The model under review builds one solid part; all positions refer to its coordinate system, in mm. A direction names the side the tool comes from. Give positions to 0.01 mm unless a question says otherwise; leave off trailing zeros. Loops run counter-clockwise (first coordinate to the right, second up) from the corner with the lowest first, then second, coordinate; pieces in that order, holes last. Notation, with made-up numbers: M 46,45 L 86,45 A15 ccw 86,74 Z; hole C 84,13 d9. An arc over 180 degrees is marked long. One line per item, written item: value. Start each with the question number.
Q1. We need section B-B on x = 1. Write out the cut boundary in (y, z), plus the area to 3 significant figures.
Q2. Mouldability with a two-part tool opening along X and no side actions: class faces 1 (the face through (4.95, 3, 0)), 2 (the face through (1, 0.2, 1.1)), 3 (the face through (4, 0, 0)) as released by +X, released by -X, zero draft, split by the parting line, or undercut.
Q3. For faces 4 (the face through (3, 4, 1.85)), 5 (the face through (-4, 0, 0)), 6 (the face through (4, 1, 1.85)), list the 3-axis set-ups (+Z, -Z, +X, -X, +Y, -Y) from which the entire face can be reached by the end or side of a thin tool; tool diameter is ignored.
Q4. We need section C-C on z = 2. Write out the cut boundary in (x, y), plus the area to 3 significant figures.
Q5. To check wall thickness, follow line 1 along Z through (x, y) = (-3, 5); line 2 along Z through (x, y) = (2.5, 2); line 3 along Z through (x, y) = (-2.25, 2.25). State the ranges of each line that lie inside material, in increasing order. Write a range as from..to.
Q6. We need section D-D on y = 4.5. Give the number of separate pieces and of enclosed holes in the cut face, plus the area to 4 significant figures.
Q7. We need section A-A on y = -0.5. Write out the cut boundary in (x, z), plus the area to 3 significant figures.
Q8. For pin 1 (0.6 mm diameter, centred on x = -3, y = -2, fed in from -Z); pin 2 (0.5 mm diameter, centred on x = 3, z = 1.5, fed in from -Y); pin 3 (2 mm diameter, centred on y = -0.5, z = 1.5, fed in from -X); pin 4 (1.5 mm diameter, centred on x = 2.5, z = -0.5, fed in from +Y), all flat-tipped, find the tip position at first contact; note any pin that passes through.
```python
from build123d import *

# Parameters (mm, degrees)
SKETCH_1_W                                 = 4.95
SKETCH_1_H                                 = 4.7
EXTRUDE_1_DEPTH                            = 1.73
EXTRUDE_2_DEPTH                            = 4.27
CUT_EXTRUDE_1_DEPTH                        = 1.5
CUT_EXTRUDE_3_DEPTH                        = 4.45
SKETCH_4_W                                 = 1.05
SKETCH_4_H                                 = 4
SKETCH_4_W_2                               = 2.45
SKETCH_4_H_2                               = 4.27
CUT_EXTRUDE_2_DEPTH                        = 0.5
CUT_EXTRUDE_4_DEPTH                        = 0.5
EXTRUDE_START                              = -5
SKETCH_5_W                                 = 0.5
SKETCH_5_H                                 = 0.5
EXTRUDE_3_DEPTH                            = 8.9
CHAMFER_1_SIZE                             = 0.1
CHAMFER_1_SIZE2                            = 0.567128182
CHAMFER_1_PART_2_SIZE                      = 0.1
CHAMFER_1_PART_2_SIZE2                     = 0.567128182
PATTERN_LINEAR_1_COUNT                     = 4
PATTERN_LINEAR_1_PITCH                     = 2
CHAMFER_1_OF_PATTERN_LINEAR_1_SIZE2        = 0.1
CHAMFER_1_OF_PATTERN_LINEAR_1_SIZE         = 0.567128182
CHAMFER_1_PART_2_OF_PATTERN_LINEAR_1_SIZE2 = 0.1
CHAMFER_1_PART_2_OF_PATTERN_LINEAR_1_SIZE  = 0.567128182


with BuildPart() as part:
    # Эскиз1 → Бобышка-Вытянуть1 (new body)
    with BuildSketch(Plane(origin=(0, 0, 0), x_dir=(1, 0, 0), z_dir=(0, 1, 0))):
        with Locations((-2.475, 0)):
            Rectangle(SKETCH_1_W, SKETCH_1_H)
    extrude_1 = extrude(amount=EXTRUDE_1_DEPTH)

    # Эскиз2 → Бобышка-Вытянуть2 (add)
    with BuildSketch(Plane(origin=(0, 1.73, 0), x_dir=(1, 0, 0), z_dir=(0, 1, 0))):
        Polygon((0, 2.35), (-4.95, 2.35), (-4.95, -2.35), (0, -2.35), (0, -1.85), (-4.45, -1.85), (-4.45, 1.85), (0, 1.85), align=None)
    extrude_2 = extrude(amount=EXTRUDE_2_DEPTH)

    # Эскиз3 → Вырез-Вытянуть1 (cut, through all)
    with BuildSketch(Plane(origin=(-4.45, 0, 0), x_dir=(0, 0, -1), z_dir=(1, 0, 0))):
        with BuildLine():
            Line((-1.35, 6), (-0.35, 6))
            Line((-0.35, 6), (-0.35, 4.3))
            ThreePointArc((-0.35, 4.3), (-0.437867966, 4.087867966), (-0.65, 4))
            Line((-0.65, 4), (-1.05, 4))
            ThreePointArc((-1.05, 4), (-1.262132034, 4.087867966), (-1.35, 4.3))
            Line((-1.35, 4.3), (-1.35, 6))
        make_face()
    cut_extrude_1 = extrude(amount=-CUT_EXTRUDE_1_DEPTH, mode=Mode.SUBTRACT)

    # Эскиз8 → Вырез-Вытянуть3 (cut)
    with BuildSketch(Plane(origin=(0, 0, 0), x_dir=(0, 0, -1), z_dir=(1, 0, 0))):
        Polygon((0, 1.73), (0.55, 1.23), (1.85, 1.23), (1.85, 1.73), align=None)
    cut_extrude_3 = extrude(amount=-CUT_EXTRUDE_3_DEPTH, mode=Mode.SUBTRACT)

    # Эскиз4 → Вырез-Вытянуть2 (cut)
    with BuildSketch(Plane.XY.offset(2.35)):
        with Locations((-3.925, 2)):
            Rectangle(SKETCH_4_W, SKETCH_4_H)
        with Locations((-1.225, 3.865)):
            Rectangle(SKETCH_4_W_2, SKETCH_4_H_2)
    cut_extrude_2 = extrude(amount=-CUT_EXTRUDE_2_DEPTH, mode=Mode.SUBTRACT)

    # Зеркальное отражение1: Бобышка-Вытянуть1, Бобышка-Вытянуть2, Вырез-Вытянуть1, Вырез-Вытянуть3, Вырез-Вытянуть2 across plane
    add(extrude_1.mirror(Plane(origin=(0, 0, 0), x_dir=(0, 0, 1), z_dir=(1, 0, 0))))
    add(extrude_2.mirror(Plane(origin=(0, 0, 0), x_dir=(0, 0, 1), z_dir=(1, 0, 0))))
    add(cut_extrude_1.mirror(Plane(origin=(0, 0, 0), x_dir=(0, 0, 1), z_dir=(1, 0, 0))), mode=Mode.SUBTRACT)
    add(cut_extrude_3.mirror(Plane(origin=(0, 0, 0), x_dir=(0, 0, 1), z_dir=(1, 0, 0))), mode=Mode.SUBTRACT)
    add(cut_extrude_2.mirror(Plane(origin=(0, 0, 0), x_dir=(0, 0, 1), z_dir=(1, 0, 0))), mode=Mode.SUBTRACT)

    # Эскиз9 → Вырез-Вытянуть4 (cut, symmetric)
    with BuildSketch(Plane.ZY.offset(3)):
        Polygon((2.35, 0), (-2.35, 0), (-2.35, 0.5), (-0.05, 0.2), (2.35, 0.2), align=None)
    cut_extrude_4 = extrude(amount=CUT_EXTRUDE_4_DEPTH, both=True, mode=Mode.SUBTRACT)

    # Эскиз5 → Бобышка-Вытянуть3 (add)
    with BuildSketch(Plane(origin=(0, 1.73, 0), x_dir=(1, 0, 0), z_dir=(0, 1, 0)).offset(EXTRUDE_START)):
        with Locations((-3, -0.65)):
            Rectangle(SKETCH_5_W, SKETCH_5_H)
    extrude_3 = extrude(amount=EXTRUDE_3_DEPTH)

    # Фаска1
    chamfer_1_edges = [part.edges().sort_by_distance(p)[0] for p in [
        (-3.25, 5.63, 0.65),
        (-3, 5.63, 0.4),
        (-2.75, 5.63, 0.65),
        (-3, 5.63, 0.9),
    ]]
    chamfer_1_side = [part.faces().sort_by_distance(p)[0] for p in [
        (-3, 5.63, 0.65),
    ]]
    chamfer(chamfer_1_edges, length=CHAMFER_1_SIZE, length2=CHAMFER_1_SIZE2, reference=chamfer_1_side[0])

    # Фаска1 part 2
    chamfer_1_part_2_edges = [part.edges().sort_by_distance(p)[0] for p in [
        (-3.25, -3.27, 0.65),
        (-3, -3.27, 0.4),
        (-2.75, -3.27, 0.65),
        (-3, -3.27, 0.9),
    ]]
    chamfer_1_part_2_side = [part.faces().sort_by_distance(p)[0] for p in [
        (-3, -3.27, 0.65),
    ]]
    chamfer(chamfer_1_part_2_edges, length=CHAMFER_1_PART_2_SIZE, length2=CHAMFER_1_PART_2_SIZE2, reference=chamfer_1_part_2_side[0])

    # Линейный массив1: Вырез-Вытянуть4, Бобышка-Вытянуть3 ×4
    with Locations(*[(i * PATTERN_LINEAR_1_PITCH, 0, 0) for i in range(1, PATTERN_LINEAR_1_COUNT)]):
        add(cut_extrude_4, mode=Mode.SUBTRACT)
        add(extrude_3)

    # Фаска1 of Линейный массив1
    chamfer_1_of_pattern_linear_1_edges = [part.edges().sort_by_distance(p)[0] for p in [
        (-1.25, 5.63, 0.65),
        (-1, 5.63, 0.4),
        (-0.75, 5.63, 0.65),
        (-1, 5.63, 0.9),
        (0.75, 5.63, 0.65),
        (1, 5.63, 0.4),
        (1.25, 5.63, 0.65),
        (1, 5.63, 0.9),
        (2.75, 5.63, 0.65),
        (3, 5.63, 0.4),
        (3.25, 5.63, 0.65),
        (3, 5.63, 0.9),
    ]]
    chamfer(chamfer_1_of_pattern_linear_1_edges, length=CHAMFER_1_OF_PATTERN_LINEAR_1_SIZE, length2=CHAMFER_1_OF_PATTERN_LINEAR_1_SIZE2)

    # Фаска1 part 2 of Линейный массив1
    chamfer_1_part_2_of_pattern_linear_1_edges = [part.edges().sort_by_distance(p)[0] for p in [
        (-1.25, -3.27, 0.65),
        (-1, -3.27, 0.4),
        (-0.75, -3.27, 0.65),
        (-1, -3.27, 0.9),
        (0.75, -3.27, 0.65),
        (1, -3.27, 0.4),
        (1.25, -3.27, 0.65),
        (1, -3.27, 0.9),
        (2.75, -3.27, 0.65),
        (3, -3.27, 0.4),
        (3.25, -3.27, 0.65),
        (3, -3.27, 0.9),
    ]]
    chamfer(chamfer_1_part_2_of_pattern_linear_1_edges, length=CHAMFER_1_PART_2_OF_PATTERN_LINEAR_1_SIZE, length2=CHAMFER_1_PART_2_OF_PATTERN_LINEAR_1_SIZE2)


solid = part.part
```
Solved:
1. outline: M -3.27,0.5 L -2.7,0.4 L 0.2,0.4 L 0.2,-0.05 L 0.5,-2.35 L 6,-2.35 L 6,-1.85 L 1.23,-1.85 L 1.23,-0.55 L 1.73,0 L 1.73,0.4 L 5.06,0.4 L 5.63,0.5 L 5.63,0.8 L 5.06,0.9 L 1.73,0.9 L 1.73,2.35 L 0.2,2.35 L 0.2,0.9 L -2.7,0.9 L -3.27,0.8 Z
1. area: 11.8 mm2
2. face 1: released by +X
2. face 2: undercut
2. face 3: zero draft
3. face 4: +Y
3. face 5: +Z, -Z, -X, -Y
3. face 6: +Z, -Y
4. outline: M -4.95,0 L -4.45,0 L -4.45,4 L -3.4,4 L -3.4,0.2 L -2.5,0.2 L -2.5,0 L -1.5,0 L -1.5,0.2 L -0.5,0.2 L -0.5,0 L 0.5,0 L 0.5,0.2 L 1.5,0.2 L 1.5,0 L 2.5,0 L 2.5,0.2 L 3.4,0.2 L 3.4,4 L 4.45,4 L 4.45,0 L 4.95,0 L 4.95,6 L 2.45,6 L 2.45,1.73 L -2.45,1.73 L -2.45,6 L -4.95,6 Z
4. area: 29.3 mm2
5. line 1: -2.35..-1.85, 0.4..0.9, 1.85..2.35
5. line 2: -2.35..-1.85, 1.85..2.35
5. line 3: -2.35..-1.85
6. separate pieces: 7
6. enclosed holes: 0
6. area: 11.15 mm2
7. outline: M -3.25,0.4 L -2.75,0.4 L -2.75,0.9 L -3.25,0.9 Z; M -1.25,0.4 L -0.75,0.4 L -0.75,0.9 L -1.25,0.9 Z; M 0.75,0.4 L 1.25,0.4 L 1.25,0.9 L 0.75,0.9 Z; M 2.75,0.4 L 3.25,0.4 L 3.25,0.9 L 2.75,0.9 Z
7. area: 1.00 mm2
8. pin 1: z = 0.4
8. pin 2: y = 0.2
8. pin 3: x = -4.95
8. pin 4: y = 1.73
